Source: CAD feature listing. Evaluate the final solid. Frame: model axes, mm. Face numbers are marked on the shaded views. A direction names the side the tool comes from. Round coordinates to 2 decimals unless told otherwise and drop trailing zeros. Order: outer loops, then holes, each group sorted by start corner. A loop starts at its lowest first (then second) coordinate and runs counter-clockwise, first axis right, second up. Notation, with made-up numbers: (50, -28) - (102, -28) arc R21 ccw to (102, 2) - close; hole circle Ø3 at (-25, 65.25). An arc over 180 degrees is marked (long way). Use one line per item in the form item = value. Start each with the question number.
Q1. Cut plane C-C, the plane z = 0.75. Return the cut outline in (x, y), and give its area (3 significant figures).
Q2. Cut plane A-A, the plane y = 0. Return the cut outline in (x, z).
Q3. Pin query (flat end, axial travel): pin 1 Ø1 at (x, z) = (2, 3) entering from -Y; pin 2 Ø1 at (y, z) = (2.5, 6.5) entering from -X; pin 3 Ø3 at (x, z) = (4, 5.5) entering from -Y. Return the tip coordinate at first contact, or that it passes through.
Q4. Ray query, line 1 (Y direction, x = 0, z = 3.75); line 2 (Z direction, x = -7, y = 0.5); line 3 (Y direction, x = 2.25, z = 3.5). Return the intervals inside material, ascending. Write a range as [from, to].
Q5. Draft query along Z for the marked faces 3, 4 and 5. Return one class per face: released by +Z, released by -Z, zero draft, split by the parting line, or undercut.
Q6. Cut plane D-D, the plane x = 2.75. Return the cut outline in (y, z).
Q7. Set-up query: the marked faces 1 and 2. Return all of +Z, -Z, +X, -X, +Y, -Y with unobstructed straight access to the full face (end or side cutting, diameter ignored); none if empty.
from build123d import *

# Parameters (mm, degrees)
SKETCH_R     = 9
PAD_DEPTH    = 9
SKETCH001_W  = 2.95
SKETCH001_H  = 7
SKETCH002_R  = 2.5
POCKET_DEPTH = 9.001


with BuildPart() as part:
    # Sketch → Pad (new body)
    with BuildSketch(Plane.XY):
        Circle(SKETCH_R)
    extrude(amount=PAD_DEPTH)

    # Sketch001 → Groove (revolve, cut)
    with BuildSketch(Plane.XZ):
        with Locations((7.525, 4.5)):
            Rectangle(SKETCH001_W, SKETCH001_H)
    revolve(axis=Axis((0, 0, 0), (0, 0, 1)), mode=Mode.SUBTRACT)

    # Sketch002 (on Face7 of Groove) → Pocket (cut, through all)
    with BuildSketch(Plane.XY.offset(9)):
        Circle(SKETCH002_R)
    extrude(amount=-POCKET_DEPTH, mode=Mode.SUBTRACT)


solid = part.part
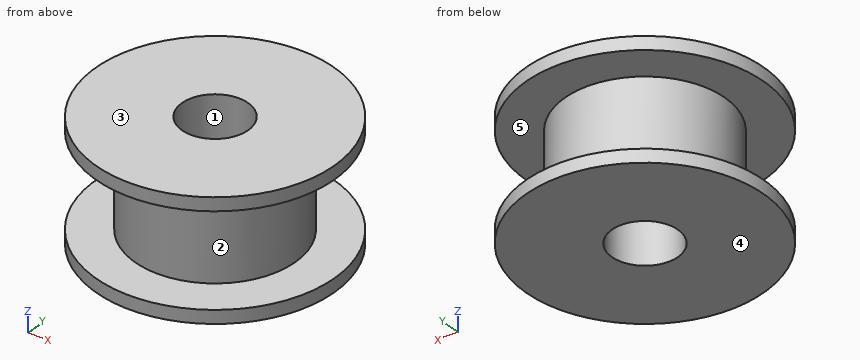
Completed:
q1.outline = circle Ø18 at (0, 0); hole circle Ø5 at (0, 0)
q1.area = 235 mm2
q2.outline = (-9, 0) - (-2.5, 0) - (-2.5, 9) - (-9, 9) - (-9, 8) - (-6.05, 8) - (-6.05, 1) - (-9, 1) - close; (2.5, 0) - (9, 0) - (9, 1) - (6.05, 1) - (6.05, 8) - (9, 8) - (9, 9) - (2.5, 9) - close
q3.pin_1 = -5.86
q3.pin_2 = -5.71
q3.pin_3 = -5.51
q4.line_1 = [-6.05, -2.5], [2.5, 6.05]
q4.line_2 = [0, 1], [8, 9]
q4.line_3 = [-5.62, -1.09], [1.09, 5.62]
q5.face_3 = released by +Z
q5.face_4 = released by -Z
q5.face_5 = undercut
q6.outline = (-8.57, 0) - (8.57, 0) - (8.57, 1) - (5.39, 1) - (5.39, 8) - (8.57, 8) - (8.57, 9) - (-8.57, 9) - (-8.57, 8) - (-5.39, 8) - (-5.39, 1) - (-8.57, 1) - close
q7.face_1 = +Z, -Z
q7.face_2 = none
